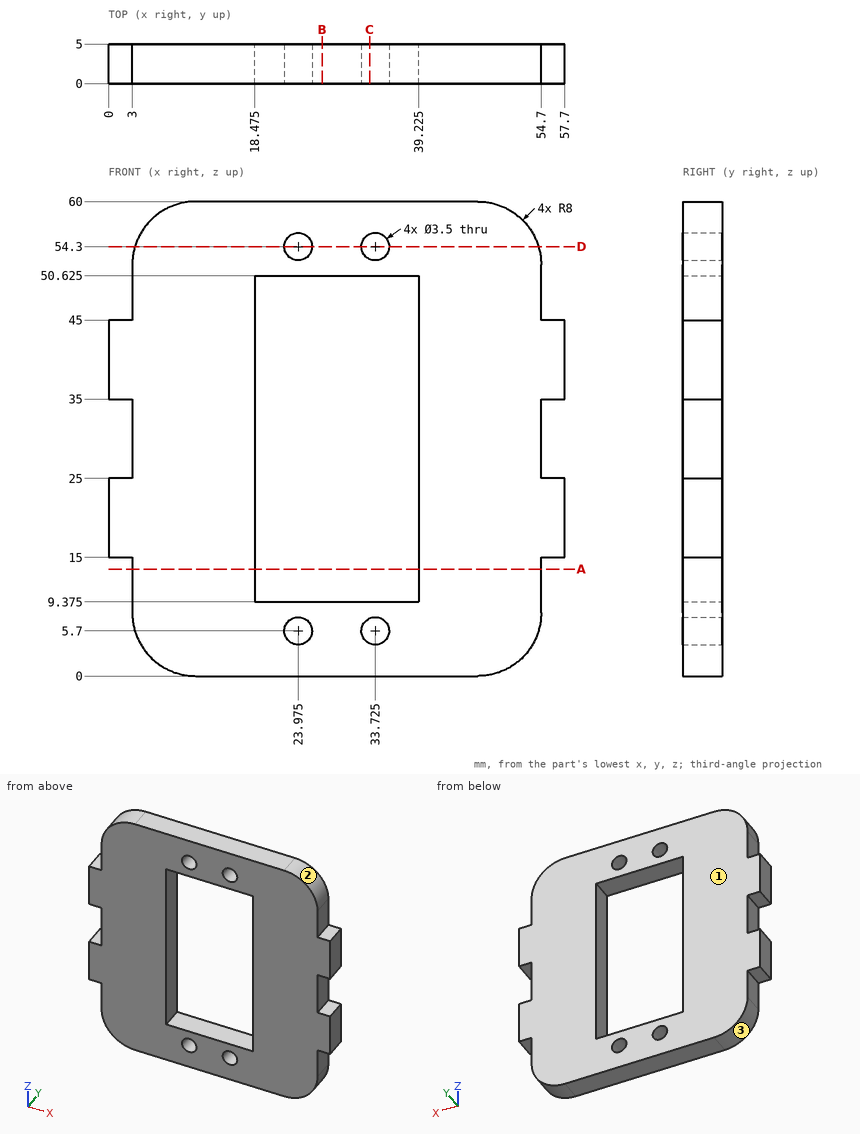
Geometry: see drawing. Coordinates: mm, zero at the bounding-box minimum. Give positions to 0.01 mm unless a question says otherwise; leave off trailing zeros. Write each loop counter-clockwise with the first axis right and the second up, starting at its lowest first coordinate (ties: lowest second). Pieces come first, ordered by that corner, then holes. Notation, with made-up numbers: (23, 75.25) - (29, 75.25) arc R24 cw to (29, 95.25) - close; hole circle Ø8 at (-5.5, -4). An arc over 180 degrees is marked (long way). Return JSON: item names as keys, results as strings. Group by question number.
1) Mould query, pull axis Z, two halves, no side actions, for the marked faces 1, 2 and 3. Classes: released by +Z, released by -Z, zero draft, split by the parting line, or undercut.
2) Section C-C on x = 33. Return the cut outline in (y, z) (3 decimals).
3) Section D-D on z = 54.3. Return the cut outline in (x, y) (3 decimals), plus the area to 3 significant figures.
4) Section B-B on x = 27. Return the cut outline in (y, z) (3 decimals), plus the area to 4 significant figures.
5) Section A-A on z = 13.5. Return the cut outline in (x, y) (3 decimals), plus the area to 3 significant figures.
6) First-contact query: P1, Ø3, axis at x = 23.975, z = 5.7, coming from the +Y side; P2, Ø0.9, axis at x = 56, y = 3, coming from the -Z side; P3, Ø1.5, axis at x = 55.5, y = 3.5, coming from the +Z side; P4, Ø1.5, axis at y = 4, z = 52, coming from the -X side. Flat tips, straight axial feed; report the tip coordinate or a pass-through.
7) Line query: line 1 (X direction, y = 3.75, z = 26) (3 decimals); line 2 (X direction, y = 3.7, z = 5.7) (3 decimals); line 3 (Z direction, x = 33, y = 3.4) (3 decimals). Output: solid intervals per line, ascending.
Filled in:
{
 "1": {"face 1": "zero draft", "face 2": "released by +Z", "face 3": "released by -Z"},
 "2": {"outline": "(0, 0) - (5, 0) - (5, 4.107) - (0, 4.107) - close; (0, 7.293) - (5, 7.293) - (5, 9.375) - (0, 9.375) - close; (0, 50.625) - (5, 50.625) - (5, 52.707) - (0, 52.707) - close; (0, 55.893) - (5, 55.893) - (5, 60) - (0, 60) - close"},
 "3": {"outline": "(3.338, 0) - (22.225, 0) - (22.225, 5) - (3.338, 5) - close; (25.725, 0) - (31.975, 0) - (31.975, 5) - (25.725, 5) - close; (35.475, 0) - (54.362, 0) - (54.362, 5) - (35.475, 5) - close", "area": "220 mm^2"},
 "4": {"outline": "(0, 0) - (5, 0) - (5, 9.375) - (0, 9.375) - close; (0, 50.625) - (5, 50.625) - (5, 60) - (0, 60) - close", "area": "93.75 mm^2"},
 "5": {"outline": "(3, 0) - (18.475, 0) - (18.475, 5) - (3, 5) - close; (39.225, 0) - (54.7, 0) - (54.7, 5) - (39.225, 5) - close", "area": "155 mm^2"},
 "6": {"P1": "passes through", "P2": "stops at z = 15", "P3": "stops at z = 45", "P4": "stops at x = 3"},
 "7": {"line 1": "x = 3 to 18.475, 39.225 to 54.7", "line 2": "x = 3.338 to 22.225, 25.725 to 31.975, 35.475 to 54.362", "line 3": "z = 0 to 4.107, 7.293 to 9.375, 50.625 to 52.707, 55.893 to 60"}
}
